from build123d import *

# Parameters (mm, degrees)
F1_DEPTH = 10
F2_ANGLE = 120
F3_W     = 10
F3_H     = 40.4382864386
F4_ANGLE = 60
F5_R     = 1


with BuildPart() as f1:
    # F0 (on Front) → F1 (new body)
    with BuildSketch(Plane.XZ):
        Polygon((0, -50), (0, 0), (-40, 0), (-40, 60), (-50, 60), (-50, -50), (-40, -50), (-40, -10), (-10, -10), (-10, -50), align=None)
    extrude(amount=F1_DEPTH)

    # F1_face (on face) → F2 (revolve)
    with BuildSketch(Plane(origin=(-31.3157894737, -10, -4.4736842105), x_dir=(1, 0, 0), z_dir=(0, -1, 0))):
        Polygon((31.3157894737, -45.5263157895), (31.3157894737, 4.4736842105), (-8.6842105263, 4.4736842105), (-8.6842105263, 64.4736842105), (-18.6842105263, 64.4736842105), (-18.6842105263, -45.5263157895), (-8.6842105263, -45.5263157895), (-8.6842105263, -5.5263157895), (21.3157894737, -5.5263157895), (21.3157894737, -45.5263157895), align=None)
    revolve(axis=Axis((0, -10, -25), (0, 0, 1)), revolution_arc=F2_ANGLE)

    # F3 (on face) → F4 (revolve, cut)
    with BuildSketch(Plane(origin=(-4.3301270189, -2.5, 0), x_dir=(-0.5, 0.8660254038, 0), z_dir=(0.8660254038, 0.5, 0))):
        with Locations((-53.6602540378, 39.7808567807)):
            Rectangle(F3_W, F3_H)
    revolve(axis=Axis((0, -10, -25), (0, 0, -1)), revolution_arc=F4_ANGLE, mode=Mode.SUBTRACT)

    # F5
    f5_edges = [f1.edges().sort_by_distance(p)[0] for p in [
        (-34.641016, -30, 60),
        (-40, -5, 60),
        (-50, -5, 60),
        (-43.30127, -35, 60),
        (-25, -53.30127, 39.780857),
        (-20, -44.641016, 39.780857),
        (-22.5, -48.971143, 60),
        (-22.5, -48.971143, 19.561714),
        (0, -50, 19.561714),
        (0, -60, 19.561714),
        (22.5, -48.971143, 19.561714),
        (10, -27.320508, 0),
        (-20, -44.641016, 0),
        (-40, -10, 30),
        (-40, -5, 0),
        (0, -5, 0),
        (25, -53.30127, -15.219143),
        (20, -44.641016, 9.780857),
        (20, -44.641016, -30),
        (12.5, -31.650635, -10),
        (5, -18.660254, -30),
        (0, -10, -25),
    ]]
    fillet(f5_edges, radius=F5_R)

    # F6: F1 across plane


with BuildPart() as f1_1:
    add(f1.part)
    add(f1.part.mirror(Plane.XZ))


solid = f1_1.part
Geometry: final body of the model. Coordinates: model frame, mm. A direction names the side the tool comes from. Give positions to 0.01 mm unless a question says otherwise; leave off trailing zeros. Order: outer loops, then holes, each group sorted by start corner. A loop starts at its lowest first (then second) coordinate and runs counter-clockwise, first axis right, second up. Notation, with made-up numbers: (-29, 66) -> (-12, 66) arc R20 cw to (-12, 102) -> close; hole circle Ø2 at (-19.5, 40.5). An arc over 180 degrees is marked (long way). Put each result on its own line as item: value.
Q1. Section D-D, the plane z = 6. Return loops of the section in (x, y), then the cut area to 3 significant figures.
Here are the results:
outline: (-50, -10) arc R50 ccw to (24.11, -53.8) arc R1 ccw to (24.49, -52.43) -> (20.49, -45.5) arc R1 ccw to (19.15, -45.12) arc R40 cw to (-40, -10) -> (-40, 10) arc R40 cw to (19.15, 45.12) arc R1 ccw to (20.49, 45.5) -> (24.49, 52.43) arc R1 ccw to (24.11, 53.8) arc R50 ccw to (-50, 10) -> close
area: 2,080 mm^2
Q2. Section B-B, the plane y = 0.5. Return loops of the section in (x, z), then the cut area to 3 significant figures.
Here are the results:
outline: (-50, -50) -> (-40, -50) -> (-40, -10) -> (-10, -10) -> (-10, -50) -> (0, -50) -> (0, -1) arc R1 ccw to (-1, 0) -> (-39, 0) arc R1 cw to (-40, 1) -> (-40, 59) arc R1 ccw to (-41, 60) -> (-49, 60) arc R1 ccw to (-50, 59) -> close
area: 1,900 mm^2
Q3. Material intervals for L1, parallel to Y at x = -6.5, z = -10.5; L2, parallel to Z at x = -20, y = 18.5; L3, parallel to Z at x = -9.5, y = 0, sorted ascending.
Here are the results:
L1: y = -59.58 to -49.47, -17.6 to 17.6, 49.47 to 59.58
L2: z = -10 to 0
L3: z = -50 to 0
Q4. Pin query (flat end, axial travel): pin 1 (16 mm diameter, centred on y = 4.5, z = 36, fed in from +X); pin 2 (1 mm diameter, centred on x = -5, y = -19.5, fed in from -Z); pin 3 (10 mm diameter, centred on x = 13.5, z = 28.5, fed in from +Y); pin 4 (1 mm diameter, centred on y = -29, z = 37.5, fed in from -X). Return the tip coordinate at first contact, or that it passes through.
Here are the results:
pin 1: stops at x = -39.92
pin 2: stops at z = -10
pin 3: passes through
pin 4: stops at x = -46.45
Q5. Section A-A, the plane z = 25.5. Return loops of the section in (x, y), then the cut area to 3 significant figures.
Here are the results:
outline: (-50, -10) arc R50 ccw to (-25.88, -52.78) arc R1 ccw to (-24.49, -52.43) -> (-20.49, -45.5) arc R1 ccw to (-20.84, -44.14) arc R40 cw to (-40, -10) -> (-40, 10) arc R40 cw to (-20.84, 44.14) arc R1 ccw to (-20.49, 45.5) -> (-24.49, 52.43) arc R1 ccw to (-25.88, 52.78) arc R50 ccw to (-50, 10) -> close
area: 1,140 mm^2
Q6. Reachability of faces 1 (the face through (-22.522, -49.01, 40.05)), 2 (the face through (12.124, 31.57, -9.699)), 3 (the face through (0, 0, -26)), 4 (the face through (-40, 0, -30)), 5 (the face through (22.2, -49.1, 19.3)) from +Z, -Z, +X, -X, +Y, -Y: full face, straight path, thin tool, end or side. Return the list, or none.
Here are the results:
face 1: +Z, +X, -Y
face 2: -Z, +X
face 3: +Z, -Z, +X
face 4: -Z
face 5: +Z, +X
Q7. Section C-C, the plane z = -33.5. Return loops of the section in (x, y), then the cut area to 3 significant figures.
Here are the results:
outline: (-50, -10) arc R50 ccw to (24.11, -53.8) arc R1 ccw to (24.49, -52.43) -> (20.49, -45.5) arc R1 ccw to (19.15, -45.12) arc R40 cw to (-40, -10) -> (-40, 10) arc R40 cw to (19.15, 45.12) arc R1 ccw to (20.49, 45.5) -> (24.49, 52.43) arc R1 ccw to (24.11, 53.8) arc R50 ccw to (-50, 10) -> close; (-10, -10) arc R10 ccw to (4.01, -19.16) arc R1 ccw to (4.47, -17.75) -> (0.13, -10.23) arc R1 cw to (0, -9.73) -> (0, 9.73) arc R1 cw to (0.13, 10.23) -> (4.47, 17.75) arc R1 ccw to (4.01, 19.16) arc R10 ccw to (-10, 10) -> close
area: 2,490 mm^2
Q8. Draft query along Y for faces 6 (the face through (-50, 0, 5)), 7 (the face through (-22.727, 48.763, 59.715)), 8 (the face through (-11, 1, 0)). Return one class per face: released by +Y, released by -Y, zero draft, split by the parting line, or undercut.
Here are the results:
face 6: zero draft
face 7: released by +Y
face 8: undercut
